Can you work these out from the model? Positions are in its coordinate system, mm. Face numbers are marked on the shaded views. Round coordinates to 2 decimals unless told otherwise and drop trailing zeros. Order: outer loops, then holes, each group sorted by start corner. A loop starts at its lowest first (then second) coordinate and runs counter-clockwise, first axis right, second up. Notation, with made-up numbers: (50.5, 8) - (58.5, 8) arc R21 cw to (58.5, 12) - close; hole circle Ø9 at (5, 73.25). An arc over 180 degrees is marked (long way). Write item = value, one per line.
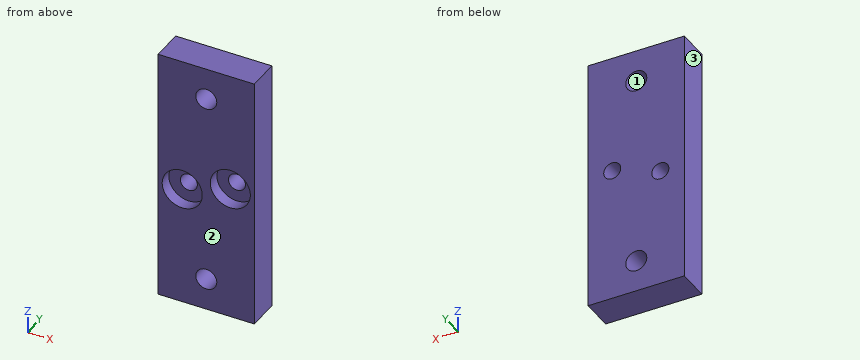
from build123d import *

# Parameters (mm, degrees)
SKETCH1_W                                    = 38.1
SKETCH1_H                                    = 101.6
SKETCH1_R                                    = 4.1656
BOSS_EXTRUDE1_DEPTH                          = 12.7
CBORE_FOR_1_4_HEX_MACHINE_SCREW1_D           = 6.7564
CBORE_FOR_1_4_HEX_MACHINE_SCREW1_CBORE_D     = 15.875
CBORE_FOR_1_4_HEX_MACHINE_SCREW1_CBORE_DEPTH = 4.826


with BuildPart() as part:
    # Sketch1 → Boss-Extrude1 (new body)
    with BuildSketch(Plane(origin=(0, 0, 0), x_dir=(1, 0, 0), z_dir=(0, 1, 0))):
        with Locations((19.05, 50.8)):
            Rectangle(SKETCH1_W, SKETCH1_H)
        with Locations(Location((19.05, 88.9, 0), (0, 0, 270))):
            Circle(SKETCH1_R, mode=Mode.SUBTRACT)
        with Locations(Location((19.05, 12.7, 0), (0, 0, 270))):
            Circle(SKETCH1_R, mode=Mode.SUBTRACT)
    extrude(amount=BOSS_EXTRUDE1_DEPTH)

    # CBORE for 1/4 Hex Machine Screw1 (through all)
    with Locations(Plane(origin=(0, 0, 0), x_dir=(-1, 0, 0), z_dir=(0, -1, 0))):
        with Locations((-28.575, 47.625), (-9.525, 53.975)):
            CounterBoreHole(CBORE_FOR_1_4_HEX_MACHINE_SCREW1_D / 2, CBORE_FOR_1_4_HEX_MACHINE_SCREW1_CBORE_D / 2, CBORE_FOR_1_4_HEX_MACHINE_SCREW1_CBORE_DEPTH)


solid = part.part
(1) If we section it at C-C (y = 1): State how many separate pieces and enclosed holes the cut face has, plus the area to 3 significant figures.
Computed:
separate_pieces = 1
enclosed_holes = 4
area = 3,370 mm^2
(2) If I drill on line 1 (Z direction, x = 28, y = 1.25); line 2 (Z direction, x = 22, y = 2.5); line 3 (X direction, y = 5.5, z = -12.7), over which ranges is the centre line in solid material (lowest first)? Write a range as from..to.
Computed:
line_1 = -101.6..-55.54, -39.71..0
line_2 = -101.6..-91.84, -85.96..-52.07, -43.18..-15.64, -9.76..0
line_3 = 0..14.88, 23.22..38.1
(3) Will this pin go through, and if not, where does the flat tip stop? P1, Ø5, axis at x = 9.5, z = -55.5, coming from the -Y side.
Computed:
P1 = 4.83
(4) Thinking about a two-plate mould opening in X: for the marked faces 1, 2 and 3, which applies, +X half, -X half, draft (parallel to the pull), parting line (faces both ways), or undercut?
Computed:
face_1 = undercut
face_2 = draft
face_3 = -X half
(5) If we section it at A-A (z = -88.9): Write out the boundary of the cut face in (x, y).
Computed:
outline = (0, 0) - (14.88, 0) - (14.88, 12.7) - (0, 12.7) - close; (23.22, 0) - (38.1, 0) - (38.1, 12.7) - (23.22, 12.7) - close
(6) If we section it at B-B (x = 19.05): Write out the boundary of the cut face in (y, z), plus the area to 3 significant figures.
Computed:
outline = (0, -101.6) - (12.7, -101.6) - (12.7, -93.07) - (0, -93.07) - close; (0, -84.73) - (12.7, -84.73) - (12.7, -16.87) - (0, -16.87) - close; (0, -8.53) - (12.7, -8.53) - (12.7, 0) - (0, 0) - close
area = 1,080 mm^2
(7) If we section it at D-D (x = 11.5): Write out the boundary of the cut face in (y, z), plus the area to 3 significant figures.
Computed:
outline = (0, -101.6) - (12.7, -101.6) - (12.7, -56.72) - (4.83, -56.72) - (4.83, -61.66) - (0, -61.66) - close; (0, -46.29) - (4.83, -46.29) - (4.83, -51.23) - (12.7, -51.23) - (12.7, 0) - (0, 0) - close
area = 1,170 mm^2
